Autodesk Inventor part; units mm, degrees
ref_plane "YZ Plane" through (0, 0, 0) normal (1, 0, 0) x (0, 1, 0)
ref_plane "XZ Plane" through (0, 0, 0) normal (0, 1, 0) x (-1, 0, 0)
ref_plane "XY Plane" through (0, 0, 0) normal (0, 0, 1) x (1, 0, 0)
sketch "Sketch1" plane through (0, 0, 0) normal (0, 0, 1) x (1, 0, 0)
  circle A0 centre (0, 0) radius 10
  circle A1 centre (-217.9737, -122.4233) radius 10
  line L0 (0, 0) -> (0, -74.3359) construction
  line L1 (-20, 0) -> (-20, -74.3359)
  line L2 (20, -74.3359) -> (20, 0)
  arc A2 (20, 0) -> (-20, 0) centre (0, 0) ccw
  arc A3 (-20, -74.3359) -> (20, -74.3359) centre (0, -74.3359) ccw
  line L3 (0, -74.3359) -> (-217.9737, -122.4233) construction
  line L4 (4.3086, -93.8662) -> (-213.6651, -141.9536)
  line L5 (-222.2823, -102.8929) -> (-4.3086, -54.8055)
  arc A4 (4.3086, -93.8662) -> (-4.3086, -54.8055) centre (0, -74.3359) ccw
  arc A5 (-222.2823, -102.8929) -> (-213.6651, -141.9536) centre (-217.9737, -122.4233) ccw
  point P0 (0, -37.1679)
  point P1 (-108.9869, -98.3796)
  dimension "d1" = 20
  dimension "d6" = 40
extrude "Extrusion1" add sketch "Sketch1" along normal blind 6
properties part number "Barra estabilizadora de ascenso"
Part model, mm, in its own coordinate system. Round coordinates to 2 decimals unless told otherwise and drop trailing zeros. Write each loop counter-clockwise with the first axis right and the second up, starting at its lowest first coordinate (ties: lowest second). Pieces come first, ordered by that corner, then holes.
Item 1: Probe L1, parallel to Y at x = 0, z = 3.2; L2, parallel to X at y = 1, z = 1.1; L3, parallel to X at y = -19.5, z = 5.4. List the from-to ranges inside material, lowest first.
Results:
L1: y = -94.82 to -10, 10 to 20
L2: x = -19.97 to -9.95, 9.95 to 19.97
L3: x = -20 to 20
Item 2: Cut at B-B, the plane z = 4.5. Give the cut face in (x, y).
Results:
outline: (-222.28, -102.89) arc R20 ccw to (-213.67, -141.95) - (4.31, -93.87) arc R20 ccw to (20, -74.34) - (20, 0) arc R20 ccw to (-20, 0) - (-20, -58.27) - close; hole circle Ø20 at (-217.97, -122.42); hole circle Ø20 at (0, 0)
Item 3: Drop flat-ended pins along their axis: pin 1 Ø12 at (x, y) = (0, 0) entering from -Z; pin 2 Ø1.8 at (y, z) = (-22, 4) entering from -X. Give the stop position or say it passes through.
Results:
pin 1: passes through
pin 2: stops at x = -20
Item 4: Cut at A-A, the plane x = 0. Give the cut face in (y, z).
Results:
outline: (-94.82, 0) - (-10, 0) - (-10, 6) - (-94.82, 6) - close; (10, 0) - (20, 0) - (20, 6) - (10, 6) - close
Item 5: Cut at D-D, the plane y = -83. Give the cut face in (x, z), plus the area to 3 significant figures.
Results:
outline: (-132.11, 0) - (18.03, 0) - (18.03, 6) - (-132.11, 6) - close
area: 901 mm2
Item 6: Two-plate mould, pull along X, no slides. Class faces 1 (the flat face through (-20, -29, 3)), 2 (the cylindrical face through (15.71, -86.71, 2.96)), 3 (the cylindrical face through (0, 20, 3)), 4 (the cylindrical face through (-219.276, -132.338, 2.958)): +X half, -X half, draft (parallel to the pull), parting line (faces both ways), or undercut.
Results:
face 1: -X half
face 2: +X half
face 3: parting line
face 4: undercut
Item 7: Cut at C-C, the plane x = -217. Give the cut face in (y, z), plus the area to 3 significant figures.
Results:
outline: (-142.4, 0) - (-132.38, 0) - (-132.38, 6) - (-142.4, 6) - close; (-112.47, 0) - (-101.73, 0) - (-101.73, 6) - (-112.47, 6) - close
area: 125 mm2
